Geometry check sheet. Reference: the model listing, model coordinates, mm. A direction names the side the tool comes from. Round coordinates to 2 decimals unless told otherwise and drop trailing zeros. Order: outer loops, then holes, each group sorted by start corner. A loop starts at its lowest first (then second) coordinate and runs counter-clockwise, first axis right, second up. Notation, with made-up numbers: (80.5, 54) - (107.5, 54) arc R24 ccw to (107.5, 83) - close; hole circle Ø5 at (-5, 64). An arc over 180 degrees is marked (long way). Return JSON: item names as keys, results as strings. Group by question number.
Q1. Draft check along X on faces 4 (the flat face through (-4.19, 69.43, 8.68)), 5 (the flat face through (-300, 63, -55)), 6 (the flat face through (-1.4, 125, -132.5)). Enter one of: pulls with the +X half, pulls with the -X half, needs draft (parallel to the pull), parting line crosses it, or undercut.
Q2. Gauge pin test, flat ends, axial feed: pin 1 Ø12 at (x, z) = (-245.5, -74.5) entering from -Y; pin 2 Ø1 at (x, y) = (205, 109.5) entering from -Z; pin 3 Ø8 at (x, z) = (-205.5, -67) entering from +Y; pin 4 Ø12 at (y, z) = (68, -14) entering from -X. Record the tip position at first contact, or that the pin passes through.
Q3. Sectioned sample at A-A, the plane y = 14.5. Record the cut outline in (x, z).
Q4. Sectioned sample at C-C, the plane x = -197. Record the cut outline in (y, z).
Q5. Sectioned sample at D-D, the plane y = 98.5. Record the cut outline in (x, z), then the cut area to 3 significant figures.
Q6. Tool access check on faces 1 (the flat face through (300, 63, -55)), 2 (the flat face through (4.2, 63.38, 9.77)), 3 (the flat face through (299, 69, -55)). Record the directions out of +Z, -Z, +X, -X, +Y, -Y that give a thin tool (end or side, any length) a straight path to the whole face; none if there is none.
Q7. Material ranges on line 1 along X through (y, z) = (120, -43.5); line 2 along X through (y, z) = (127.5, -104.5); line 3 along X through (y, z) = (55, -119.5), recorded low to high.
Q8. Sectioned sample at B-B, the plane z = -64. Record the cut outline in (x, y), then the cut area to 3 significant figures.
```python
from build123d import *

# Parameters (mm, degrees)
BOSS_EXTRUDE1_DEPTH = 300
SKETCH2_W           = 616.91666666
SKETCH2_H           = 169.999999994
BOSS_EXTRUDE2_DEPTH = 5
CUT_EXTRUDE1_START  = -300
CUT_EXTRUDE1_DEPTH  = 299


with BuildPart() as part:
    # Sketch1 → Boss-Extrude1 (new, symmetric)
    with BuildSketch(Plane(origin=(0, 0, 0), x_dir=(0, 0, -1), z_dir=(1, 0, 0))):
        Polygon((0, 0), (113, 0), (133.041666667, 130), (-20.041666667, 130), align=None)
    extrude(amount=BOSS_EXTRUDE1_DEPTH, both=True)

    # Sketch2 → Boss-Extrude2 (add, symmetric)
    with BuildSketch(Plane(origin=(0, 130, 0), x_dir=(1, 0, 0), z_dir=(0, 1, 0))):
        with Locations((0, 56.5)):
            Rectangle(SKETCH2_W, SKETCH2_H)
    extrude(amount=BOSS_EXTRUDE2_DEPTH, both=True)

    # Sketch3 → Cut-Extrude1 (cut, symmetric)
    with BuildSketch(Plane.ZY.offset(300).offset(CUT_EXTRUDE1_START)):
        Polygon((-131.788872207, 135), (18.788872207, 135), (-1.71529446, 2), (-111.28470554, 2), align=None)
    extrude(amount=CUT_EXTRUDE1_DEPTH, both=True, mode=Mode.SUBTRACT)


solid = part.part
```
Reply:
{
 "1": {"face 4": "undercut", "face 5": "pulls with the -X half", "face 6": "needs draft"},
 "2": {"pin 1": "y = 0", "pin 2": "z = -129.96", "pin 3": "y = 2", "pin 4": "x = -300"},
 "3": {"outline": "(-300, -115.24) - (300, -115.24) - (300, 2.24) - (-300, 2.24) - close; hole (-299, -113.21) - (299, -113.21) - (299, 0.21) - (-299, 0.21) - close"},
 "4": {"outline": "(0, -113) - (125, -132.27) - (125, -141.5) - (135, -141.5) - (135, -131.79) - (2, -111.28) - (2, -1.72) - (135, 18.79) - (135, 28.5) - (125, 28.5) - (125, 19.27) - (0, 0) - close"},
 "5": {"outline": "(-300, -128.19) - (300, -128.19) - (300, 15.19) - (-300, 15.19) - close; hole (-299, -126.16) - (299, -126.16) - (299, 13.16) - (-299, 13.16) - close", "area": "2,710 mm^2"},
 "6": {"face 1": "+Z, -Z, +X, -Y", "face 2": "+Z, +X, -X, -Y", "face 3": "+Y"},
 "7": {"line 1": "-300 to -299, 299 to 300", "line 2": "-308.46 to -299, 299 to 308.46", "line 3": "-300 to 300"},
 "8": {"outline": "(-308.46, 125) - (-300, 125) - (-300, 0) - (300, 0) - (300, 125) - (308.46, 125) - (308.46, 135) - (299, 135) - (299, 2) - (-299, 2) - (-299, 135) - (-308.46, 135) - close", "area": "1,640 mm^2"}
}
